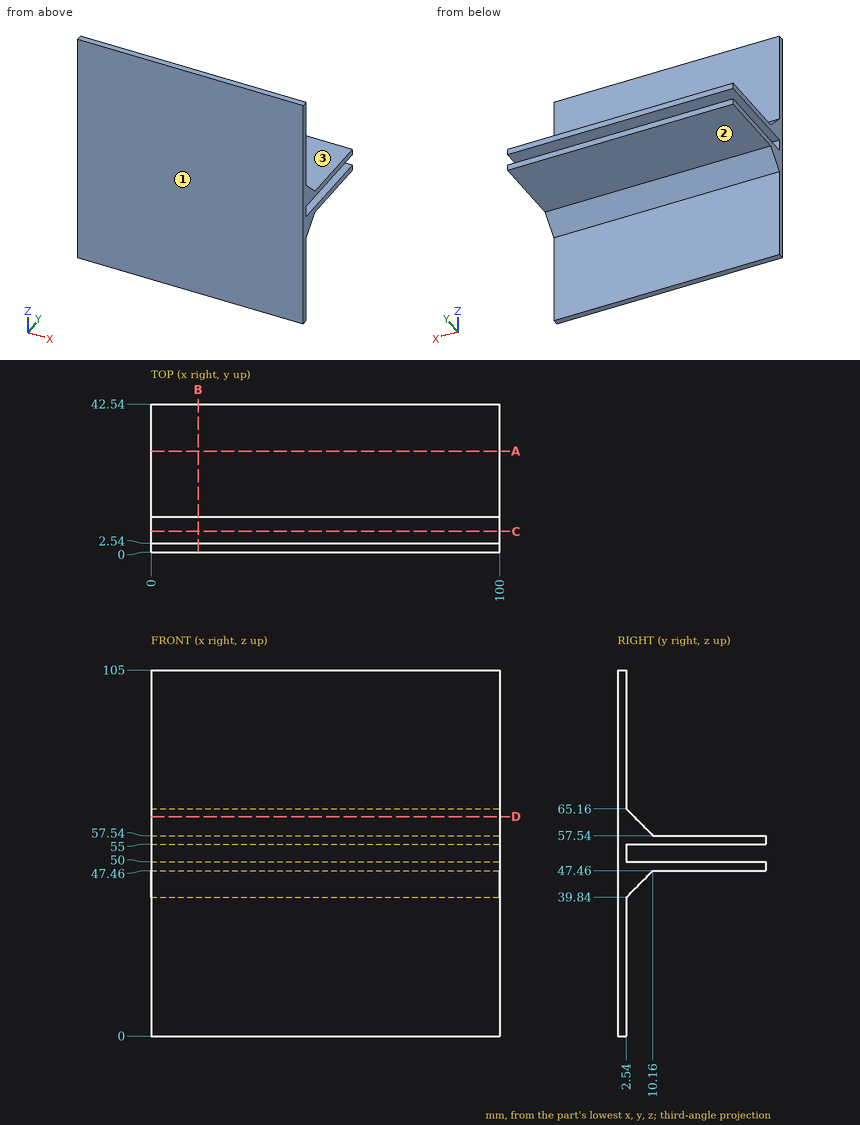
Design review of the part shown in the three views and the two pictorial views. Dimensions are in mm from the part's minimum x, y and z. A direction names the side the tool comes from. Give positions to 0.01 mm unless a question says otherwise; leave off trailing zeros. Write each loop counter-clockwise with the first axis right and the second up, starting at its lowest first coordinate (ties: lowest second). Pieces come first, ordered by that corner, then holes.
Item 1: Take a section at C-C (y = 6). Give the boundary of the cut face in (x, z).
Item 2: Wall thickness on probe 1 along Z at (x, y) = (57, 22.5); probe 2 along Y at (x, z) = (78.5, 6); probe 3 along Z at (x, y) = (30, 4.5): over which ranges is each line inside the solid? List them lowest first.
Item 3: Machinability: for the marked faces 1, 2 and 3, which of the approach directions +Z, -Z, +X, -X, +Y, -Y give a long, thin tool a straight path to every point of the face, cutting with its end or side? Answer none if there is none.
Item 4: Take a section at D-D (z = 63). Give the boundary of the cut face in (x, y), and give its area (3 significant figures).
Item 5: Take a section at A-A (y = 29). Give the boundary of the cut face in (x, z), and give its area (3 significant figures).
Item 6: Take a section at B-B (x = 13.5). Give the boundary of the cut face in (y, z).
Item 7: Insertion check: P1, Ø1, axis at x = 11.5, y = 9.5, coming from the +Z side; P2, Ø1.5, axis at x = 73, z = 51.5, coming from the +Y side; P3, Ø3, axis at x = 53.5, y = 21.5, coming from the +Z side. Each pin has a flat end and moves straight along its axis. Give the tip position at first contact, or say it passes through.
Established:
1. outline: (0, 43.3) - (100, 43.3) - (100, 50) - (0, 50) - close; (0, 55) - (100, 55) - (100, 61.7) - (0, 61.7) - close
2. probe 1: z = 47.46 to 50, 55 to 57.54
2. probe 2: y = 0 to 2.54
2. probe 3: z = 41.8 to 50, 55 to 63.2
3. face 1: +Z, -Z, +X, -X, -Y
3. face 2: -Z, +X, -X, +Y
3. face 3: +Z, +X, -X, +Y
4. outline: (0, 0) - (100, 0) - (100, 4.7) - (0, 4.7) - close
4. area: 470 mm2
5. outline: (0, 47.46) - (100, 47.46) - (100, 50) - (0, 50) - close; (0, 55) - (100, 55) - (100, 57.54) - (0, 57.54) - close
5. area: 508 mm2
6. outline: (0, 0) - (2.54, 0) - (2.54, 39.84) - (10.16, 47.46) - (42.54, 47.46) - (42.54, 50) - (2.54, 50) - (2.54, 55) - (42.54, 55) - (42.54, 57.54) - (10.16, 57.54) - (2.54, 65.16) - (2.54, 105) - (0, 105) - close
7. P1: stops at z = 58.7
7. P2: stops at y = 2.54
7. P3: stops at z = 57.54
